Verification items for this drawing (mm, ordinates from the low corner). A direction names the side the tool comes from. Give positions to 0.01 mm unless a question says otherwise; leave off trailing zeros. Loops run counter-clockwise (first coordinate to the right, second up) from the corner with the lowest first, then second, coordinate; pieces in that order, holes last. Notation, with made-up numbers: M 84,33.25 L 107,33.25 A23 cw 107,68.25 Z; hole C 35.5,-28.5 d7. An arc over 180 degrees is marked long. Use a Markdown table: item, result.
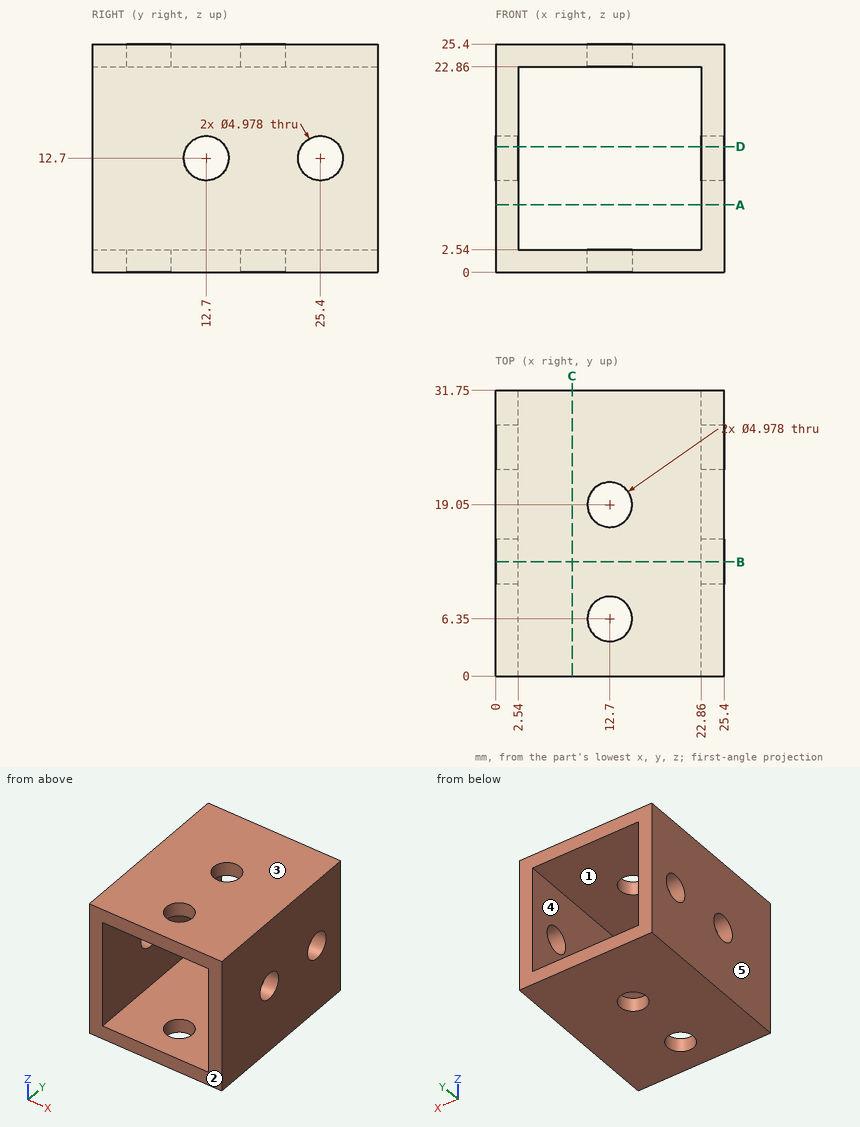
(1) Cross-section at C-C on x = 8.5. Record the cut outline in (y, z), then the cut area to 3 significant figures.
Results below:
| item | result |
|---|---|
| outline | M 0,0 L 31.75,0 L 31.75,2.54 L 0,2.54 Z; M 0,22.86 L 31.75,22.86 L 31.75,25.4 L 0,25.4 Z |
| area | 161 mm^2 |
(2) Material ranges on line 1 (Y direction, x = 12.7, z = 1.3); line 2 (X direction, y = 8.5, z = 11.5), recorded low to high.
Results below:
| item | result |
|---|---|
| line 1 | 0 to 3.86, 8.84 to 16.56, 21.54 to 31.75 |
| line 2 | 0 to 2.54, 22.86 to 25.4 |
(3) Cross-section at D-D on z = 14. Record the cut outline in (x, y).
Results below:
| item | result |
|---|---|
| outline | M 0,0 L 2.54,0 L 2.54,10.58 L 0,10.58 Z; M 0,14.82 L 2.54,14.82 L 2.54,23.28 L 0,23.28 Z; M 0,27.52 L 2.54,27.52 L 2.54,31.75 L 0,31.75 Z; M 22.86,0 L 25.4,0 L 25.4,10.58 L 22.86,10.58 Z; M 22.86,14.82 L 25.4,14.82 L 25.4,23.28 L 22.86,23.28 Z; M 22.86,27.52 L 25.4,27.52 L 25.4,31.75 L 22.86,31.75 Z |
(4) Draft check along X on the marked faces 3, 4 and 5. Enter one of: +X half, -X half, draft (parallel to the pull), parting line (faces both ways), or undercut.
Results below:
| item | result |
|---|---|
| face 3 | draft |
| face 4 | undercut |
| face 5 | -X half |
(5) Cross-section at B-B on y = 12.7. Record the cut outline in (x, z), then the cut area to 3 significant figures.
Results below:
| item | result |
|---|---|
| outline | M 0,0 L 25.4,0 L 25.4,10.21 L 22.86,10.21 L 22.86,2.54 L 2.54,2.54 L 2.54,10.21 L 0,10.21 Z; M 0,15.19 L 2.54,15.19 L 2.54,22.86 L 22.86,22.86 L 22.86,15.19 L 25.4,15.19 L 25.4,25.4 L 0,25.4 Z |
| area | 207 mm^2 |
(6) Cross-section at A-A on z = 7.5. Record the cut outline in (x, y), then the cut area to 3 significant figures.
Results below:
| item | result |
|---|---|
| outline | M 0,0 L 2.54,0 L 2.54,31.75 L 0,31.75 Z; M 22.86,0 L 25.4,0 L 25.4,31.75 L 22.86,31.75 Z |
| area | 161 mm^2 |
(7) Set-up check for the marked faces 1 and 2: record each of +Z, -Z, +X, -X, +Y, -Y from which the full face is reachable in a straight line by a thin tool's end or side.
Results below:
| item | result |
|---|---|
| face 1 | +Y, -Y |
| face 2 | +Z, -Z, +X, -X, -Y |
